Geometry check sheet. Reference: drawing and pictorial views, mm from the part's lowest x, y, z. Round coordinates to 2 decimals unless told otherwise and drop trailing zeros. Order: outer loops, then holes, each group sorted by start corner. A loop starts at its lowest first (then second) coordinate and runs counter-clockwise, first axis right, second up.
(1) Sectioned sample at A-A (x = 6.75). Record the boundary of the cut face in (y, z).
(2) Sectioned sample at B-B (y = 2.5). Record the boundary of the cut face in (x, z), plus the area to 3 significant figures.
(3) Material ranges on line 1 along X through (y, z) = (1.7, 1.4); line 2 along X through (y, z) = (0.9, 2.4); line 3 along Z through (x, y) = (9, 2.8), recorded low to high.
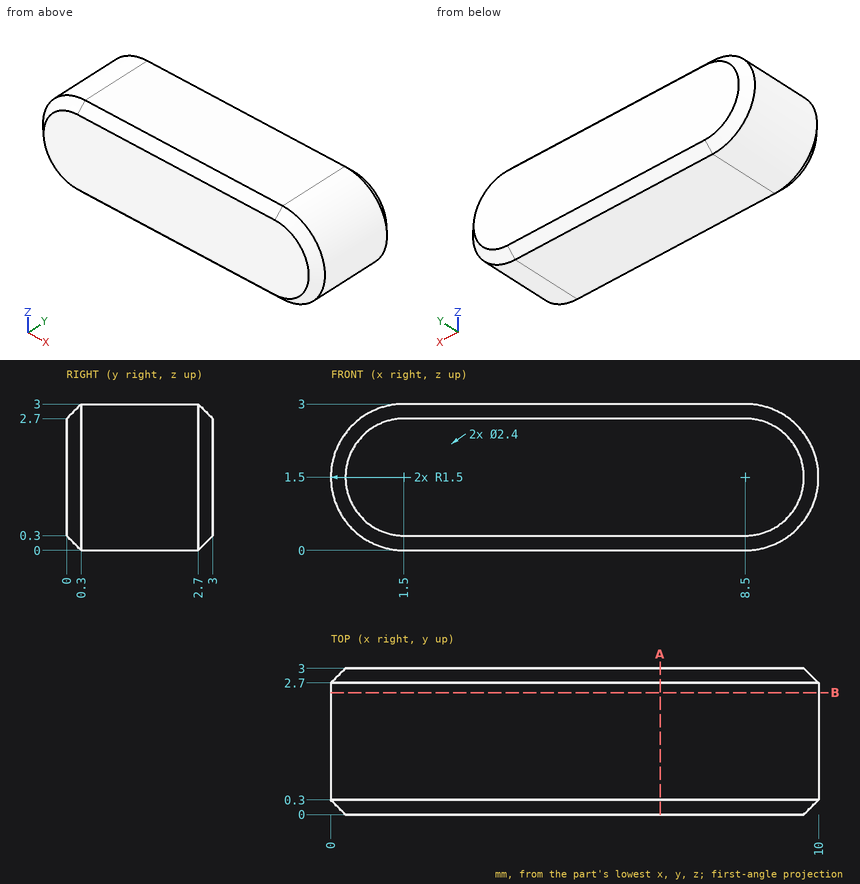
Answer below:
1. outline: (0, 0.3) - (0.3, 0) - (2.7, 0) - (3, 0.3) - (3, 2.7) - (2.7, 3) - (0.3, 3) - (0, 2.7) - close
2. outline: (1.5, 0) - (8.5, 0) arc R1.5 ccw to (8.5, 3) - (1.5, 3) arc R1.5 ccw to start
2. area: 28.1 mm2
3. line 1: x = 0 to 10
3. line 2: x = 0.3 to 9.7
3. line 3: z = 0.19 to 2.81
